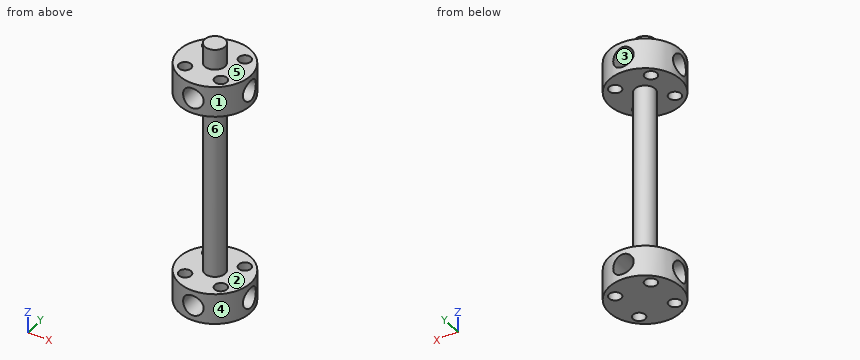
Autodesk Inventor part; units mm, degrees
ref_plane "Work Plane2" through (0, 11.1125, 0) normal (0, 1, 0) x (-1, 0, 0)
ref_plane "YZ Plane" through (0, 0, 0) normal (1, 0, 0) x (0, 1, 0)
ref_plane "XY Plane" through (0, 0, 0) normal (0, 0, 1) x (1, 0, 0)
sketch "Sketch2" plane through (0, 0, 0) normal (0, 0, 1) x (1, 0, 0)
  line L0 (0, 0) -> (3.175, -3.175)
  circle A0 centre (0, 0) radius 11.1125
  dimension "d6" = 22.225
extrude "Extrusion2" add sketch "Sketch2" along normal mid plane 9.525
sketch "Sketch6" plane through (0, 0, 4.7625) normal (0, 0, 1) x (1, 0, 0)
  circle A0 centre (0, 0) radius 3.175
  dimension "d17" = 6.35
extrude "Extrusion3" add sketch "Sketch6" along normal blind 28.448
sketch "Sketch7" plane through (0, 0, 4.7625) normal (0, 0, 1) x (1, 0, 0)
  circle A0 centre (0, 0) radius 3.175
  line L0 (5.8251, 5.4849) -> (0.0652, -0.2751)
  line L1 (0, 0) -> (5.491, 0)
  dimension "d20" = 8.001
  dimension "d42" = 45
hole "Hole2" at (5.8251, 5.4849, 4.7625) direction (0, 0, -1) diameter 3.81 end through all
pattern_circular "Circular Pattern2" count 4 over 360 about axis through (0, 0, 4.7625) along (0, 0, 1) of "Hole2"
ref_plane "Work Plane2" through (0, 11.1125, 0) normal (0, 1, 0) x (-1, 0, 0)
sketch "Sketch8" plane through (0, 11.1125, 0) normal (0, 1, 0) x (-1, 0, 0)
  point P0 (0, 0)
  point P1 (0, 0)
hole "Hole3" at (0, 11.1125, 0) direction (0, -1, 0) diameter 6.35 end through all
pattern_circular "Circular Pattern3" count 4 over 360 about axis through (0, 0, 4.7625) along (0, 0, 1) of "Hole3"
mirror "Mirror1" about plane through (0, 0, 33.2105) normal (0, 0, 1) of "Extrusion2", "Hole2", "Circular Pattern2", "Extrusion3", "Hole3", "Circular Pattern3"
sketch "Sketch9" plane through (0, 0, 71.1835) normal (0, 0, 1) x (1, 0, 0)
  line L0 (0, 0) -> (0, 0)
  circle A0 centre (0, 0) radius 3.175
  dimension "d43" = 6.35
extrude "Extrusion4" add sketch "Sketch9" along normal blind 6.35
properties part number "SweeperHub"
Can you work these out from the model? Positions are in its coordinate system, mm. Face numbers are marked on the shaded views. A direction names the side the tool comes from. Give positions to 0.01 mm unless a question says otherwise; leave off trailing zeros. Loops run counter-clockwise (first coordinate to the right, second up) from the corner with the lowest first, then second, coordinate; pieces in that order, holes last. Notation, with made-up numbers: M 2,16 L 55,16 A11 ccw 55,31 Z; hole C 17,52 d6. An arc over 180 degrees is marked long. Answer in a Markdown table with one row per item.
1. For pin 1 Ø4 at (x, y) = (-1.5, 5) entering from +Z; pin 2 Ø6 at (x, z) = (6.5, 68.5) entering from +Y; pin 3 Ø4 at (y, z) = (-7, 32) entering from -X; pin 4 Ø6 at (x, z) = (2.5, 12.5) entering from +Y (3 decimals), each with a flat end and sliding along its axis, tell me the tip position at first contact or that it passes through.
Taken from the geometry:
| item | result |
|---|---|
| pin 1 | stops at z = 71.18 |
| pin 2 | stops at y = 10.55 |
| pin 3 | passes through |
| pin 4 | stops at y = 3.175 |
2. Suppose I cut it at A-A on x = -9.5. Count the separate pieces of the cut face and the enclosed holes in it, plus the area to 3 significant figures.
Taken from the geometry:
| item | result |
|---|---|
| separate pieces | 2 |
| enclosed holes | 2 |
| area | 156 mm² |
3. Thinking about a two-plate mould opening in X: for the marked faces 1, 2 and 3, which applies, released by +X, released by -X, zero draft, split by the parting line, or undercut?
Taken from the geometry:
| item | result |
|---|---|
| face 1 | split by the parting line |
| face 2 | zero draft |
| face 3 | undercut |
4. Which directions (+Z, -Z, +X, -X, +Y, -Y) give clear straight access to the entire face, cutting with the end or side of a thin tool? Please do the marked faces 4, 5 and 6.
Taken from the geometry:
| item | result |
|---|---|
| face 4 | +Z, -Z |
| face 5 | +Z |
| face 6 | none |
5. Suppose I cut it at C-C on z = 0. Write out the boundary of the cut face in (x, y) (1 decimal), plus the area to 3 significant figures.
Taken from the geometry:
| item | result |
|---|---|
| outline | M -10.6,-3.2 A11.1 ccw -3.2,-10.6 L -3.2,-3.2 Z; M -10.6,3.2 L -3.2,3.2 L -3.2,10.6 A11.1 ccw Z; M 3.2,-10.6 A11.1 ccw 10.6,-3.2 L 3.2,-3.2 Z; M 3.2,3.2 L 10.6,3.2 A11.1 ccw 3.2,10.6 Z; hole C -5.8,-5.5 d3.8; hole C -5.5,5.8 d3.8; hole C 5.5,-5.8 d3.8; hole C 5.8,5.5 d3.8 |
| area | 104 mm² |
6. If I drill on line 1 along Z through (x, y) = (0, -2.5) (1 decimal); line 2 along Z through (x, y) = (3.5, 0) (1 decimal); line 3 along Z through (x, y) = (0.25, 0.75), over which ranges is the centre line in solid material (lowest first)?
Taken from the geometry:
| item | result |
|---|---|
| line 1 | z = -4.8 to -3.2, 3.2 to 63.2, 69.6 to 77.5 |
| line 2 | z = -4.8 to -3.2, 3.2 to 4.8, 61.7 to 63.2, 69.6 to 71.2 |
| line 3 | z = -4.76 to -3.17, 3.17 to 63.26, 69.59 to 77.53 |
